from build123d import *

# Parameters (mm, degrees)
SKETCH1_W                = 82
SKETCH1_H                = 150
BOSS_EXTRUDE1_DEPTH      = 10
SKETCH2_W                = 10
SKETCH2_H                = 45
BOSS_EXTRUDE2_DEPTH      = 82
BOSS_EXTRUDE3_DEPTH      = 42
BOSS_EXTRUDE3_DEPTH_BACK = 10
FILLET3_RADIUS           = 26
FILLET3_LENGTH           = 10
FILLET4_RADIUS           = 26
FILLET4_LENGTH           = 10
BOSS_EXTRUDE4_DEPTH      = 10
BOSS_EXTRUDE5_DEPTH      = 10
FILLET5_R                = 15
FILLET6_R                = 15
SKETCH6_R                = 8
SKETCH6_R_2              = 5.5
CUT_EXTRUDE1_DEPTH       = 131.057679512
FILLET7_R                = 3
FILLET8_R                = 3
FILLET9_R                = 3
FILLET10_R               = 3
FILLET11_R               = 2
SKETCH7_R                = 5.5
CUT_EXTRUDE2_DEPTH       = 116.043470045
SKETCH8_W                = 181.068808942
SKETCH8_H                = 99.289789265
CUT_EXTRUDE3_DEPTH       = 126.678160394
SKETCH9_W                = 17.116284166
SKETCH9_H                = 92.331504729
BOSS_EXTRUDE6_DEPTH      = 10
SKETCH10_W               = 23.658167423
SKETCH10_H               = 25.148445686
SKETCH10_W_2             = 13.971358715
SKETCH10_H_2             = 14.716497846
BOSS_EXTRUDE7_DEPTH      = 10


with BuildPart() as part:
    # Sketch1 → Boss-Extrude1 (new body)
    with BuildSketch(Plane(origin=(0, 0, 0), x_dir=(1, 0, 0), z_dir=(0, 1, 0))):
        Rectangle(SKETCH1_W, SKETCH1_H)
    extrude(amount=BOSS_EXTRUDE1_DEPTH)

    # Sketch2 → Boss-Extrude2 (add, through all)
    with BuildSketch(Plane(origin=(41, 0, 0), x_dir=(0, 0, -1), z_dir=(1, 0, 0))):
        with Locations((70, 22.5)):
            Rectangle(SKETCH2_W, SKETCH2_H)
    extrude(amount=-BOSS_EXTRUDE2_DEPTH)

    # Sketch3 → Boss-Extrude3 (add, two sides: drawn at the far end of the back side and taken through both)
    with BuildSketch(Plane.XY.offset(-65).offset(-BOSS_EXTRUDE3_DEPTH_BACK)):
        Polygon((10, 45), (10, 10), (20, 10), (20, 45), (20, 87), (10, 87), align=None)
        Polygon((-10, 45), (-10, 87), (-20, 87), (-20, 45), (-20, 10), (-10, 10), align=None)
    extrude(amount=BOSS_EXTRUDE3_DEPTH + BOSS_EXTRUDE3_DEPTH_BACK)

    # Fillet3: full round fillet: the end face becomes a half cylinder, R = half its width
    fillet3_face = Plane((15, 87, -49), x_dir=(-1, 0, 0), z_dir=(0, 1, 0))  # on the end face: x along it, z out of the body
    fillet3_slab = fillet3_face.offset(-FILLET3_RADIUS / 2) * Box(FILLET3_LENGTH, 2 * FILLET3_RADIUS, FILLET3_RADIUS, mode=Mode.PRIVATE)  # the body's end, R deep
    fillet3_round = Plane((15, 61, -49), x_dir=(0, 1, 0), z_dir=(-1, 0, 0)) * Cylinder(FILLET3_RADIUS, FILLET3_LENGTH, mode=Mode.PRIVATE)  # its axis R under the face
    add(fillet3_slab - fillet3_round, mode=Mode.SUBTRACT)

    # Fillet4: full round fillet: the end face becomes a half cylinder, R = half its width
    fillet4_face = Plane((-15, 87, -49), x_dir=(-1, 0, 0), z_dir=(0, 1, 0))  # on the end face: x along it, z out of the body
    fillet4_slab = fillet4_face.offset(-FILLET4_RADIUS / 2) * Box(FILLET4_LENGTH, 2 * FILLET4_RADIUS, FILLET4_RADIUS, mode=Mode.PRIVATE)  # the body's end, R deep
    fillet4_round = Plane((-15, 61, -49), x_dir=(0, 1, 0), z_dir=(-1, 0, 0)) * Cylinder(FILLET4_RADIUS, FILLET4_LENGTH, mode=Mode.PRIVATE)  # its axis R under the face
    add(fillet4_slab - fillet4_round, mode=Mode.SUBTRACT)

    # Sketch4 → Boss-Extrude4 (add)
    with BuildSketch(Plane(origin=(20, 0, 0), x_dir=(0, 0, -1), z_dir=(1, 0, 0))):
        Polygon((23, 10), (23, 50), (-75, 25), (-75, 10), align=None)
    extrude(amount=-BOSS_EXTRUDE4_DEPTH)

    # Sketch5 → Boss-Extrude5 (add)
    with BuildSketch(Plane.ZY.offset(20)):
        Polygon((-23, 50), (75, 25), (75, 10), (-23, 10), align=None)
    extrude(amount=-BOSS_EXTRUDE5_DEPTH)

    # Fillet5
    fillet5_edges = [part.edges().sort_by_distance(p)[0] for p in [
        (15, 25, 75),
    ]]
    fillet(fillet5_edges, radius=FILLET5_R)

    # Fillet6
    fillet6_edges = [part.edges().sort_by_distance(p)[0] for p in [
        (-15, 25, 75),
    ]]
    fillet(fillet6_edges, radius=FILLET6_R)

    # Sketch6 → Cut-Extrude1 (cut, through all)
    with BuildSketch(Plane(origin=(20, 0, 0), x_dir=(0, 0, -1), z_dir=(1, 0, 0))):
        with Locations((49, 61)):
            Circle(SKETCH6_R)
        with Locations((-60, 17.5)):
            Circle(SKETCH6_R_2)
    extrude(amount=-CUT_EXTRUDE1_DEPTH, mode=Mode.SUBTRACT)

    # Fillet7
    fillet7_edges = [part.edges().sort_by_distance(p)[0] for p in [
        (30.5, 45, -65),
    ]]
    fillet(fillet7_edges, radius=FILLET7_R)

    # Fillet8
    fillet8_edges = [part.edges().sort_by_distance(p)[0] for p in [
        (0, 45, -65),
    ]]
    fillet(fillet8_edges, radius=FILLET8_R)

    # Fillet9
    fillet9_edges = [part.edges().sort_by_distance(p)[0] for p in [
        (-30.5, 45, -65),
    ]]
    fillet(fillet9_edges, radius=FILLET9_R)

    # Fillet10
    fillet10_edges = [part.edges().sort_by_distance(p)[0] for p in [
        (30.5, 10, -65),
        (0, 10, -65),
        (-30.5, 10, -65),
    ]]
    fillet(fillet10_edges, radius=FILLET10_R)

    # Fillet11
    fillet11_edges = [part.edges().sort_by_distance(p)[0] for p in [
        (15, 50, -23),
        (-15, 50, -23),
    ]]
    fillet(fillet11_edges, radius=FILLET11_R)

    # Sketch7 → Cut-Extrude2 (cut, through all)
    with BuildSketch(Plane(origin=(0, 10, 0), x_dir=(1, 0, 0), z_dir=(0, 1, 0))):
        with Locations(Location((31.5, 45, 0), (0, 0, 270))):
            Circle(SKETCH7_R)
        with Locations(Location((31.5, -15, 0), (0, 0, 270))):
            Circle(SKETCH7_R)
        with Locations(Location((-31.5, -15, 0), (0, 0, 90))):
            Circle(SKETCH7_R)
        with Locations(Location((-31.5, 45, 0), (0, 0, 90))):
            Circle(SKETCH7_R)
    extrude(amount=-CUT_EXTRUDE2_DEPTH, mode=Mode.SUBTRACT)

    # Sketch8 → Cut-Extrude3 (cut, through all)
    with BuildSketch(Plane.ZY.offset(-10)):
        with Locations((1.490278263, 42.723870649)):
            Rectangle(SKETCH8_W, SKETCH8_H)
    extrude(amount=CUT_EXTRUDE3_DEPTH, mode=Mode.SUBTRACT)

    # Sketch9 → Boss-Extrude6 (add, through all)
    with BuildSketch(Plane(origin=(0, 10, 0), x_dir=(1, 0, 0), z_dir=(0, 1, 0))):
        with Locations((30.200951285, 11.209960756)):
            Rectangle(SKETCH9_W, SKETCH9_H)
    extrude(amount=-BOSS_EXTRUDE6_DEPTH)

    # Sketch10 → Boss-Extrude7 (add)
    with BuildSketch(Plane.ZY.offset(-10)):
        with Locations((-48.340901153, 61.662766329)):
            Rectangle(SKETCH10_W, SKETCH10_H)
        with Locations((59.331703342, 16.768133659)):
            Rectangle(SKETCH10_W_2, SKETCH10_H_2)
    extrude(amount=-BOSS_EXTRUDE7_DEPTH)


solid = part.part
Check sheet for the modelled part. Datum: model origin and axes. Units: mm. A direction names the side the tool comes from. Coordinates: 2 decimals unless noted, no trailing zeros. Loops run counter-clockwise (first coordinate to the right, second up) from the corner with the lowest first, then second, coordinate; pieces in that order, holes last. Notation, with made-up numbers: (59.5, 40.5) -> (79.5, 40.5) arc R17 cw to (79.5, 61.5) -> close; hole circle Ø4 at (83.25, -26.75). An arc over 180 degrees is marked (long way). Write item = value, one per line. Start each with the question number.
1. Material ranges on line 1 (Y direction, x = 35, z = 69.5); line 2 (X direction, y = 73, z = -45.5); line 3 (Z direction, x = 38.5, y = 32.5), recorded low to high.
2. Tool access check on faces 1 (the flat face through (15, 56, -23)), 2 (the cylindrical face through (30.35, 44.1, -65.86)), 3 (the flat face through (31, 45, -71)), 4 (the flat face through (25, 0, -1)). Record the directions out of +Z, -Z, +X, -X, +Y, -Y that give a thin tool (end or side, any length) a straight path to the whole face; none if there is none.
3. Depth check by flat-ended pin: P1, Ø6.5, axis at x = 35.5, y = 22, coming from the +Z side; P2, Ø3, axis at x = 21, y = 53, coming from the +Z side; P3, Ø5, axis at x = 27, z = -54.5, coming from the +Y side. Enter the tip coordinate at first touch or a pass-through.
4. Section check D-D on x = 13. Record the cut outline in (y, z).
5. Section check B-B on z = -49. Record the cut outline in (x, y).
6. Section check A-A on x = 25. Record the cut outline in (y, z), then the cut area to 3 significant figures.
7. Section check C-C on y = 17.5. Record the cut outline in (x, z).
Responses:
q1.line_1 = 0 to 10
q1.line_2 = 10 to 20
q1.line_3 = -75 to -65
q2.face_1 = +Z, +X, -X, +Y
q2.face_2 = +Z, +X, +Y
q2.face_3 = +Z, -Z, +X, +Y
q2.face_4 = +Z, -Z, +X, -X, -Y
q3.P1 = -65
q3.P2 = -23
q3.P3 = 10
q4.outline = (0, -75) -> (61, -75) arc R26 ccw to (61, -23) -> (51.55, -23) arc R2 cw to (49.62, -21.49) -> (27.88, 63.71) arc R15 ccw to (13.35, 75) -> (0, 75) -> close
q5.outline = (10, 0) -> (41, 0) -> (41, 10) -> (20, 10) -> (20, 87) -> (10, 87) -> close
q6.outline = (0, -75) -> (45, -75) -> (45, -68) arc R3 ccw to (42, -65) -> (13, -65) arc R3 cw to (10, -62) -> (10, 75) -> (0, 75) -> close
q6.area = 1,850 mm2
q7.outline = (10, -75) -> (41, -75) -> (41, -65) -> (20, -65) -> (20, 74.41) -> (10, 74.41) -> close
